Source: CAD feature listing. Evaluate the final solid. Frame: model axes, mm. A direction names the side the tool comes from. Give positions to 0.01 mm unless a question says otherwise; leave off trailing zeros. Loops run counter-clockwise (first coordinate to the right, second up) from the corner with the lowest first, then second, coordinate; pieces in that order, holes last. Notation, with made-up numbers: M 77,53.5 L 119,53.5 A13 ccw 119,67.5 Z; hole C 74,68.5 d7. An arc over 180 degrees is marked long. Answer in a Markdown table with one row per item.
```python
from build123d import *

# Parameters (mm, degrees)
SKETCH1_W           = 762
SKETCH1_H           = 165.1
BOSS_EXTRUDE1_DEPTH = 2.38125
SKETCH2_W           = 762
SKETCH2_H           = 50.8
BOSS_EXTRUDE2_DEPTH = 6.35
SKETCH3_W           = 762
SKETCH3_H           = 25.4
CUT_EXTRUDE1_DEPTH  = 6.35
SKETCH4_W           = 6.35
SKETCH4_H           = 165.1
BOSS_EXTRUDE3_DEPTH = 6.35


with BuildPart() as part:
    # Sketch1 → Boss-Extrude1 (new body)
    with BuildSketch(Plane(origin=(0, 0, 0), x_dir=(1, 0, 0), z_dir=(0, 1, 0))):
        Rectangle(SKETCH1_W, SKETCH1_H)
    extrude(amount=BOSS_EXTRUDE1_DEPTH)

    # Sketch2 → Boss-Extrude2 (add)
    with BuildSketch(Plane(origin=(0, 2.38125, 0), x_dir=(1, 0, 0), z_dir=(0, 1, 0))):
        with Locations((0, 44.45)):
            Rectangle(SKETCH2_W, SKETCH2_H)
    extrude(amount=BOSS_EXTRUDE2_DEPTH)

    # Sketch3 → Cut-Extrude1 (cut)
    with BuildSketch(Plane(origin=(0, 8.73125, 0), x_dir=(1, 0, 0), z_dir=(0, 1, 0))):
        with Locations((0, 44.45)):
            Rectangle(SKETCH3_W, SKETCH3_H)
    extrude(amount=-CUT_EXTRUDE1_DEPTH, mode=Mode.SUBTRACT)

    # Sketch4 → Boss-Extrude3 (add)
    with BuildSketch(Plane(origin=(0, 2.38125, 0), x_dir=(1, 0, 0), z_dir=(0, 1, 0))):
        with Locations((-377.825, 0)):
            Rectangle(SKETCH4_W, SKETCH4_H)
    extrude(amount=BOSS_EXTRUDE3_DEPTH)


solid = part.part
```
1) Section A-A, the plane x = -327.5. Return loops of the section in (y, z).
Reply:
| item | result |
|---|---|
| outline | M 0,-82.55 L 2.38,-82.55 L 2.38,-69.85 L 8.73,-69.85 L 8.73,-57.15 L 2.38,-57.15 L 2.38,-31.75 L 8.73,-31.75 L 8.73,-19.05 L 2.38,-19.05 L 2.38,82.55 L 0,82.55 Z |
2) Section C-C, the plane y = 5.75. Return loops of the section in (x, z).
Reply:
| item | result |
|---|---|
| outline | M -381,-82.55 L -374.65,-82.55 L -374.65,-69.85 L 381,-69.85 L 381,-57.15 L -374.65,-57.15 L -374.65,-31.75 L 381,-31.75 L 381,-19.05 L -374.65,-19.05 L -374.65,82.55 L -381,82.55 Z |
3) Material intervals for L1, parallel to Z at x = -52.5, y = 3; L2, parallel to Y at x = -126, z = -50; L3, parallel to X at y = 6.25, z = -51, sorted ascending.
Reply:
| item | result |
|---|---|
| L1 | z = -69.85 to -57.15, -31.75 to -19.05 |
| L2 | y = 0 to 2.38 |
| L3 | x = -381 to -374.65 |
4) Set-up query: faces 3 (the flat face through (-5, 0, -1)), 4 (the flat face through (-2, 2.381, -76)). Return all of +Z, -Z, +X, -X, +Y, -Y with unobstructed straight access to the full face (end or side cutting, diameter ignored); none if empty.
Reply:
| item | result |
|---|---|
| face 3 | +Z, -Z, +X, -X, -Y |
| face 4 | -Z, +X, +Y |
5) Pin query (flat end, axial travel): pin 1 Ø5 at (y, z) = (6, -77) entering from +X; pin 2 Ø4 at (x, z) = (-122, -77.5) entering from +Y; pin 3 Ø12 at (x, z) = (-198.5, -10) entering from -Y; pin 4 Ø1 at (x, y) = (-256.5, 3) entering from -Z. Return the tip coordinate at first contact, or that it passes through.
Reply:
| item | result |
|---|---|
| pin 1 | stops at x = -374.65 |
| pin 2 | stops at y = 2.38 |
| pin 3 | stops at y = 0 |
| pin 4 | stops at z = -69.85 |
6) Pull-direction query (Z, two-part tool) for faces 1 (the flat face through (-2, 2.381, 31)), 2 (the flat face through (-2, 2.381, -45)); classes: released by +Z, released by -Z, zero draft, split by the parting line, or undercut.
Reply:
| item | result |
|---|---|
| face 1 | zero draft |
| face 2 | undercut |
7) Section B-B, the plane z = 24.5. Return loops of the section in (x, y).
Reply:
| item | result |
|---|---|
| outline | M -381,0 L 381,0 L 381,2.38 L -374.65,2.38 L -374.65,8.73 L -381,8.73 Z |
